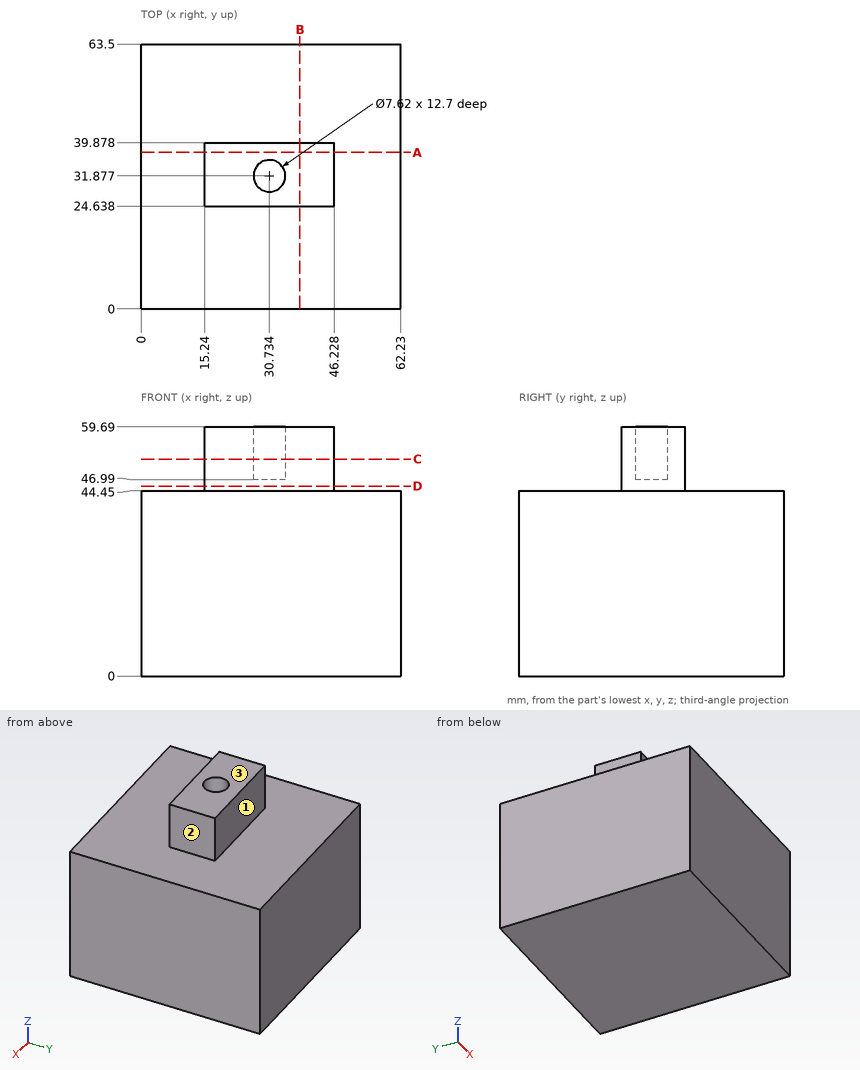
Could you check a few things on this drawing? It's one solid part, dimensions in mm from its lowest x, y, z. A direction names the side the tool comes from. Give positions to 0.01 mm unless a question says otherwise; leave off trailing zeros. Write each loop counter-clockwise with the first axis right and the second up, starting at its lowest first coordinate (ties: lowest second). Pieces come first, ordered by that corner, then holes. Notation, with made-up numbers: M -5,25 L 26,25 A25 ccw 26,43 Z; hole C -16,-38 d1. An arc over 180 degrees is marked long. Put each result on its own line as item: value. Start each with the question number.
Item 1: If we section it at C-C, the plane z = 52: Write out the boundary of the cut face in (x, y), then the cut area to 3 significant figures.
Item 2: Will these pins go through, and if not, where does the flat tip stop? pin 1 (8 mm diameter, centred on x = 10, y = 36.5, fed in from +Z); pin 2 (4.5 mm diameter, centred on y = 31.5, z = 53.5, fed in from +X); pin 3 (17 mm diameter, centred on x = 29.5, z = 55, fed in from -Y).
Item 3: On a 3-axis mill with a long thin cutter (end or side, diameter ignored), from which of +Z, -Z, +X, -X, +Y, -Y can I reach the whole of each face in a straight line? I mean the marked faces 1, 2 and 3. Say none if no direction works.
Item 4: I need wall thicknesses on L1, parallel to Z at x = 25.5, y = 56.5; L2, parallel to X at y = 26.5, z = 54; L3, parallel to Y at x = 43.5, z = 53. Which ranges of each line are inside material? Lowest first, please. Write a range as from..to.
Item 5: If we section it at B-B, the plane x = 38: Write out the boundary of the cut face in (y, z), then the cut area to 3 significant figures.
Item 6: If we section it at D-D, the plane z = 45.5: Write out the boundary of the cut face in (x, y).
Item 7: If we section it at A-A, the plane y = 37.5: Write out the boundary of the cut face in (x, z).
Values:
1. outline: M 15.24,24.64 L 46.23,24.64 L 46.23,39.88 L 15.24,39.88 Z; hole C 30.73,31.88 d7.62
1. area: 427 mm²
2. pin 1: z = 44.45
2. pin 2: x = 46.23
2. pin 3: y = 24.64
3. face 1: +Z, +X, -X, +Y
3. face 2: +Z, +X, +Y, -Y
3. face 3: +Z, +X, -X, +Y, -Y
4. L1: 0..44.45
4. L2: 15.24..46.23
4. L3: 24.64..39.88
5. outline: M 0,0 L 63.5,0 L 63.5,44.45 L 39.88,44.45 L 39.88,59.69 L 24.64,59.69 L 24.64,44.45 L 0,44.45 Z
5. area: 3,050 mm²
6. outline: M 15.24,24.64 L 46.23,24.64 L 46.23,39.88 L 15.24,39.88 Z
7. outline: M 0,0 L 62.23,0 L 62.23,44.45 L 46.23,44.45 L 46.23,59.69 L 15.24,59.69 L 15.24,44.45 L 0,44.45 Z
